For this review, take the finished solid that the model builds, in its own axes (mm). A direction names the side the tool comes from. Give positions to 0.01 mm unless a question says otherwise; leave off trailing zeros. Order: outer loops, then holes, each group sorted by start corner. A loop starts at its lowest first (then second) coordinate and runs counter-clockwise, first axis right, second up. Notation, with made-up numbers: (28, 56) -> (80, 56) arc R18 cw to (80, 91) -> close; hole circle Ø9 at (-3.75, -36). An arc over 180 degrees is marked (long way). Use CSV: the item, a comma, the result in double quotes. Start each with the question number.
```python
from build123d import *

# Parameters (mm, degrees)
SKETCH1_W           = 25.4
SKETCH1_H           = 12.7
BOSS_EXTRUDE1_DEPTH = 17.78
SKETCH2_W           = 3.175
SKETCH2_H           = 12.7
CUT_EXTRUDE1_DEPTH  = 16.51
SKETCH3_R           = 1.5875
BOSS_EXTRUDE2_DEPTH = 3.175
CUT_EXTRUDE2_DEPTH  = 23.753920541


with BuildPart() as part:
    # Sketch1 → Boss-Extrude1 (new body)
    with BuildSketch(Plane(origin=(0, 0, 0), x_dir=(1, 0, 0), z_dir=(0, 1, 0))):
        Rectangle(SKETCH1_W, SKETCH1_H)
    extrude(amount=BOSS_EXTRUDE1_DEPTH)

    # Sketch2 → Cut-Extrude1 (cut)
    with BuildSketch(Plane.XZ):
        with Locations((-11.1125, 0)):
            Rectangle(SKETCH2_W, SKETCH2_H)
        with Locations((11.1125, 0)):
            Rectangle(SKETCH2_W, SKETCH2_H)
    extrude(amount=-CUT_EXTRUDE1_DEPTH, mode=Mode.SUBTRACT)

    # Sketch3 → Boss-Extrude2 (add)
    with BuildSketch(Plane(origin=(0, 17.78, 0), x_dir=(1, 0, 0), z_dir=(0, 1, 0))):
        with Locations(Location((-5.08, 0, 0), (0, 0, 90))):
            Circle(SKETCH3_R)
    extrude(amount=BOSS_EXTRUDE2_DEPTH)

    # Sketch4 → Cut-Extrude2 (cut, through all)
    with BuildSketch(Plane(origin=(0, 17.78, 0), x_dir=(1, 0, 0), z_dir=(0, 1, 0))):
        with BuildLine():
            Line((-11.43, -4.445), (-12.7, -4.445))
            Line((-12.7, -4.445), (-12.7, -1.905))
            Line((-12.7, -1.905), (-11.43, -1.905))
            ThreePointArc((-11.43, -1.905), (-10.16, -3.175), (-11.43, -4.445))
        make_face()
        with BuildLine():
            Line((-11.43, 1.905), (-12.7, 1.905))
            Line((-12.7, 1.905), (-12.7, 4.445))
            Line((-12.7, 4.445), (-11.43, 4.445))
            ThreePointArc((-11.43, 4.445), (-10.16, 3.175), (-11.43, 1.905))
        make_face()
        with BuildLine():
            Line((12.7, 4.445), (11.43, 4.445))
            ThreePointArc((11.43, 4.445), (10.16, 3.175), (11.43, 1.905))
            Line((11.43, 1.905), (12.7, 1.905))
            Line((12.7, 1.905), (12.7, 4.445))
        make_face()
        with BuildLine():
            Line((12.7, -1.905), (11.43, -1.905))
            ThreePointArc((11.43, -1.905), (10.16, -3.175), (11.43, -4.445))
            Line((11.43, -4.445), (12.7, -4.445))
            Line((12.7, -4.445), (12.7, -1.905))
        make_face()
    extrude(amount=-CUT_EXTRUDE2_DEPTH, mode=Mode.SUBTRACT)


solid = part.part
```
1. Consider section D-D (z = 3.5). State the section outline as (x, y) points (3 decimals).
2. For faces 4 (the face through (-4.114, 19.345, 1.26)), 5 (the face through (11, 16.51, 0)), 6 (the face through (12, 17, -1.905)), list the 3-axis set-ups (+Z, -Z, +X, -X, +Y, -Y) from which the entire face can be reached by the end or side of a thin tool; tool diameter is ignored.
3. Consider section B-B (z = 0). State the section outline as (x, y) points (1 decimal), plus the area to 3 significant figures.
4. Draft analysis for pull direction Z (two halves, no side actions). For faces 1 (the face through (12, 17, -4.445)), 2 (the face through (-12.7, 17, -5)), 3 (the face through (0, 9, -6.35)), state which applies: +Z half, -Z half, draft (parallel to the pull), parting line (faces both ways), or undercut.
5. To check wall thickness, follow L1, parallel to X at y = 11.75, z = 2.5 (3 decimals); L2, parallel to Y at x = 5, z = 1.5; L3, parallel to Y at x = -10, z = -5.5. State the ranges of each line that lie inside material, in increasing order. Write a range as [from, to].
6. Clearance check with flat-ended pins moving along their axes: P1, Ø6.5, axis at y = 9.5, z = 2, coming from the +X side (3 decimals); P2, Ø6.5, axis at y = 10, z = -0.5, coming from the -X side (3 decimals); P3, Ø1.5, axis at x = 0, z = 3, coming from the +Y side. State where each tip first meets the part, or that it passes through.
7. Consider section C-C (y = 7.75). State the section outline as (x, z) points (3 decimals).
Answer list:
1,outline,"(-10.202, 16.51) -> (-9.525, 16.51) -> (-9.525, 0) -> (9.525, 0) -> (9.525, 16.51) -> (10.202, 16.51) -> (10.202, 17.78) -> (-10.202, 17.78) -> close"
2,face 4,"+Y"
2,face 5,"+Z, -Z, +X, -Y"
2,face 6,"+X, +Y, -Y"
3,outline,"(-12.7, 16.5) -> (-9.5, 16.5) -> (-9.5, 0) -> (9.5, 0) -> (9.5, 16.5) -> (12.7, 16.5) -> (12.7, 17.8) -> (-3.5, 17.8) -> (-3.5, 21) -> (-6.7, 21) -> (-6.7, 17.8) -> (-12.7, 17.8) -> close"
3,area,"357 mm2"
4,face 1,"undercut"
4,face 2,"draft"
4,face 3,"-Z half"
5,L1,"[-9.525, 9.525]"
5,L2,"[0, 17.78]"
5,L3,"[16.51, 17.78]"
6,P1,"x = 9.525"
6,P2,"x = -9.525"
6,P3,"y = 17.78"
7,outline,"(-9.525, -6.35) -> (9.525, -6.35) -> (9.525, 6.35) -> (-9.525, 6.35) -> close"
